Geometry check sheet. Reference: the model listing, model coordinates, mm. A direction names the side the tool comes from. Round coordinates to 2 decimals unless told otherwise and drop trailing zeros. Order: outer loops, then holes, each group sorted by start corner. A loop starts at its lowest first (then second) coordinate and runs counter-clockwise, first axis right, second up. Notation, with made-up numbers: M 55.5,46.5 L 69.5,46.5 A22 ccw 69.5,83.5 Z; hole C 34,63.25 d5. An arc over 180 degrees is marked long. Answer as a JSON object with one key per item and string values. Group by question number.
```python
from build123d import *

# Parameters (mm, degrees)
RESSALTO_EXTRUS_O1_DEPTH = 10


with BuildPart() as part:
    # Esboço1 → Ressalto-extrusão1 (new body)
    with BuildSketch(Plane.XY):
        Polygon((0, 0), (0, 15), (-8.675387099, 9.084963341), (-4.450360915, 2.88825827), (-5.689701929, 2.043253033), (-9.914728114, 8.239958104), (-22, 0), align=None)
    extrude(amount=RESSALTO_EXTRUS_O1_DEPTH)


solid = part.part
```
1) Sectioned sample at B-B (y = 7). Record the boundary of the cut face in (x, z).
2) Sectioned sample at D-D (x = -3.5). Record the boundary of the cut face in (y, z).
3) Go/stop test with a flat-tipped pin: P1, Ø1, axis at x = -12, z = 4.5, coming from the +Y side. Record where the tip stops, or that it passes through.
4) Sectioned sample at A-A (x = -6). Record the boundary of the cut face in (y, z).
5) Thickness scan on line 1 along X through (y, z) = (5.5, 3.5); line 2 along X through (y, z) = (2.5, 5.5); line 3 along Y through (x, z) = (-7, 1.25). Record the ranges inside material, lowest first. Write a range as [from, to].
6) Release check for a two-part mould opening along Y. For faces 3 (the flat face through (-15.87, 4.18, 4.93)), 4 (the flat face through (-7.773, 5.098, 4.93)), 5 (the flat face through (-11, 0, 5)) record: +Y half, -Y half, draft (parallel to the pull), parting line (faces both ways), or undercut.
7) Sectioned sample at C-C (z = 6.5). Record the boundary of the cut face in (x, y), then the cut area to 3 significant figures.
8) Set-up check for faces 1 (the flat face through (-6.592, 6.03, 4.93)), 2 (the flat face through (-4.28, 12.08, 4.93)): record each of +Z, -Z, +X, -X, +Y, -Y from which the full face is reachable in a straight line by a thin tool's end or side.
Final values:
{
 "1": {"outline": "M -11.73,0 L -9.07,0 L -9.07,10 L -11.73,10 Z; M -7.25,0 L 0,0 L 0,10 L -7.25,10 Z"},
 "2": {"outline": "M 0,0 L 12.61,0 L 12.61,10 L 0,10 Z"},
 "3": {"P1": "stops at y = 7.16"},
 "4": {"outline": "M 0,0 L 2.5,0 L 2.5,10 L 0,10 Z; M 5.16,0 L 10.91,0 L 10.91,10 L 5.16,10 Z"},
 "5": {"line 1": "x = [-13.93, -8.05], [-6.23, 0]", "line 2": "x = [-18.33, -6], [-5.02, 0]", "line 3": "y = [0, 3.97], [6.63, 10.23]"},
 "6": {"face 3": "+Y half", "face 4": "undercut", "face 5": "-Y half"},
 "7": {"outline": "M -22,0 L 0,0 L 0,15 L -8.68,9.08 L -4.45,2.89 L -5.69,2.04 L -9.91,8.24 Z", "area": "154 mm^2"},
 "8": {"face 1": "+Z, -Z", "face 2": "+Z, -Z, -X, +Y"}
}
